Geometry check sheet. Reference: the model listing, model coordinates, mm. A direction names the side the tool comes from. Coordinates: 2 decimals unless noted, no trailing zeros. Loops run counter-clockwise (first coordinate to the right, second up) from the corner with the lowest first, then second, coordinate; pieces in that order, holes last. Notation, with made-up numbers: (4.25, 53.25) - (24.25, 53.25) arc R24 cw to (24.25, 77.25) - close; hole circle Ø10 at (-4.5, 65). An arc over 180 degrees is marked (long way). One line per item, written item: value.
from build123d import *

# Parameters (mm, degrees)
F1_DEPTH = 10
F2_R     = 7
F3_DEPTH = 2
F4_R     = 5
F5_DEPTH = 36
F6_W     = 1.5
F6_H     = 1.416463
F8_R     = 5
F9_DEPTH = 22


with BuildPart() as f1:
    # F0 (on Right) → F1 (new body)
    with BuildSketch(Plane.YZ):
        Polygon((-6.350853, -11), (6.350853, -11), (12.701706, 0), (6.350853, 11), (-6.350853, 11), (-12.701706, 0), align=None)
    extrude(amount=-F1_DEPTH)

    # F2 (on face) → F3 (join)
    with BuildSketch(Plane.YZ):
        Circle(F2_R)
    extrude(amount=F3_DEPTH)

    # F4 (on face) → F5 (join)
    with BuildSketch(Plane.YZ.offset(2)):
        Circle(F4_R)
    extrude(amount=F5_DEPTH)

    # F6 (on Front) → F7 (revolve, cut)
    with BuildSketch(Plane.XZ):
        with Locations((34.95, -4.708232)):
            Rectangle(F6_W, F6_H)
    revolve(axis=Axis((38, 0, 0), (1, 0, 0)), mode=Mode.SUBTRACT)

    # F8 (on face) → F9 (join)
    with BuildSketch(Plane(origin=(-10, 0, 0), x_dir=(0, -1, 0), z_dir=(-1, 0, 0))):
        Circle(F8_R)
    extrude(amount=F9_DEPTH)


solid = f1.part
(1) Cross-section at A-A on y = 0. Record the cut outline in (x, z), and give its area (3 significant figures).
Reply:
outline: (-32, -5) - (-10, -5) - (-10, -11) - (0, -11) - (0, -7) - (2, -7) - (2, -5) - (34.2, -5) - (34.2, -4) - (35.7, -4) - (35.7, -5) - (38, -5) - (38, 5) - (35.7, 5) - (35.7, 4) - (34.2, 4) - (34.2, 5) - (2, 5) - (2, 7) - (0, 7) - (0, 11) - (-10, 11) - (-10, 5) - (-32, 5) - close
area: 825 mm2
(2) Go/stop test with flat-tipped pins: pin 1 Ø1 at (y, z) = (1.5, 7) entering from +X; pin 2 Ø1.5 at (x, y) = (23, -4.5) entering from +Z; pin 3 Ø6 at (y, z) = (9.5, -4.5) entering from -X. Record where each tip stops, or that it passes through.
Reply:
pin 1: x = 2
pin 2: z = 3.31
pin 3: x = -10
(3) Cross-section at C-C on z = 3. Record the cut outline in (x, y), and give its area (3 significant figures).
Reply:
outline: (-32, -4) - (-10, -4) - (-10, -10.97) - (0, -10.97) - (0, -6.32) - (2, -6.32) - (2, -4) - (34.2, -4) - (34.2, -2.65) - (35.7, -2.65) - (35.7, -4) - (38, -4) - (38, 4) - (35.7, 4) - (35.7, 2.65) - (34.2, 2.65) - (34.2, 4) - (2, 4) - (2, 6.32) - (0, 6.32) - (0, 10.97) - (-10, 10.97) - (-10, 4) - (-32, 4) - close
area: 705 mm2
(4) Material ranges on probe 1 along X at (y, z) = (1.25, -4); probe 2 along X at (y, z) = (-2.5, 5.75); probe 3 along X at (y, z) = (10.75, 0), recorded low to high. Write a range as from..to.
Reply:
probe 1: -32..34.2, 35.7..38
probe 2: -10..2
probe 3: -10..0
(5) Cross-section at D-D on y = -8.25. Record the cut outline in (x, z), and give its area (3 significant figures).
Reply:
outline: (-10, -7.71) - (0, -7.71) - (0, 7.71) - (-10, 7.71) - close
area: 154 mm2
(6) Cross-section at B-B on x = 7. Record the cut outline in (y, z).
Reply:
outline: circle Ø10 at (0, 0)
(7) Access from +Z, -Z, +X, -X, +Y, -Y to the whole of each face (thin tool, end or side, straight path). Record for faces 5 (the face through (-20.85, 1.08, -4.88)), 6 (the face through (0.986, 6.466, -2.681)), 7 (the face through (-4.93, -9.48, 5.58)).
Reply:
face 5: -X
face 6: +X
face 7: +Z, +X, -X, -Y
(8) Release check for a two-part mould opening along X. For faces 1 (the face through (-5, 0, -11)), 2 (the face through (2, -2, 5)), 3 (the face through (35, -2.4, 3.2)), 4 (the face through (-10, 5.5, 0.2)) record: pulls with the +X half, pulls with the -X half, needs draft (parallel to the pull), parting line crosses it, or undercut.
Reply:
face 1: needs draft
face 2: pulls with the +X half
face 3: undercut
face 4: pulls with the -X half
